Input: part model. Units: mm. Frame: model coordinates. Face numbers are marked on the shaded views. A direction names the side the tool comes from. Give positions to 0.01 mm unless a question says otherwise; leave off trailing zeros. Loops run counter-clockwise (first coordinate to the right, second up) from the corner with the lowest first, then second, coordinate; pieces in that order, holes last. Notation, with made-up numbers: M 27,53.5 L 63,53.5 A26 cw 63,70.5 Z; hole C 16.5,-19 d10. An arc over 180 degrees is marked long. Use CSV: the item, a comma, the result in double quotes. Start each with the question number.
Q1. Section D-D, the plane x = 29. Output: boundary loops of the cut face in (y, z), plus the area to 3 significant figures.
Q2. Reachability of the marked faces 1, 2, 3, 4 and 5 from +Z, -Z, +X, -X, +Y, -Y: full face, straight path, thin tool, end or side. Return the list, or none.
Q3. Pin query (flat end, axial travel): pin 1 (1.5 mm diameter, centred on x = 13, y = 65.5, fed in from +Z); pin 2 (5.5 mm diameter, centred on x = -23, z = 23, fed in from -Y); pin 3 (4 mm diameter, centred on y = 48, z = 26, fed in from +X). Return the tip coordinate at first contact, or that it passes through.
Q4. Section A-A, the plane y = 65. State how many separate pieces and enclosed holes the cut face has, plus the area to 3 significant figures.
Q5. Pull-direction query (Y, two-part tool) for the marked faces 6, 7, 8 and 9; classes: released by +Y, released by -Y, zero draft, split by the parting line, or undercut.
Q6. Section B-B, the plane x = -3. Output: boundary loops of the cut face in (y, z), plus the area to 3 significant figures.
Q7. Material intervals for line 1 along X through (y, z) = (24, 32); line 2 along Z through (x, y) = (28.5, 34); line 3 along X through (y, z) = (3.75, -23), sorted ascending.
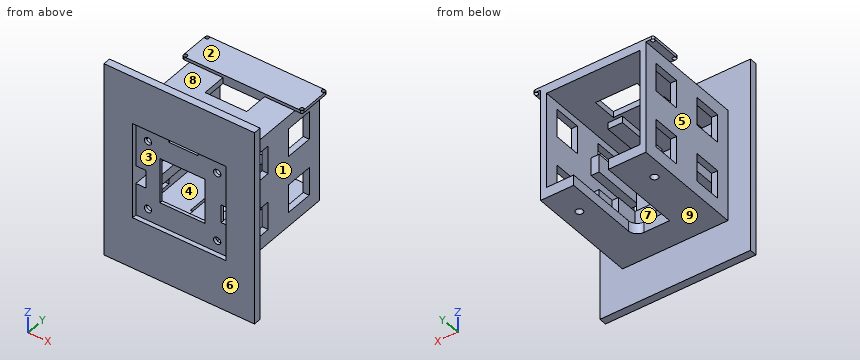
from build123d import *

# Parameters (mm, degrees)
SKETCH_1_W           = 100
SKETCH_1_H           = 130
EXTRUDE_1_DEPTH      = 5
SKETCH_2_W           = 70
SKETCH_2_H           = 75
SKETCH_2_W_2         = 62
SKETCH_2_H_2         = 64
EXTRUDE_2_DEPTH      = 73.5
SKETCH_3_W           = 18.75
SKETCH_3_H           = 18.4
CUT_EXTRUDE_1_DEPTH  = 133.711152508
CUT_EXTRUDE_2_DEPTH  = 10
SKETCH_7_W           = 62
SKETCH_7_H           = 64
CUT_EXTRUDE_3_DEPTH  = 3
SKETCH_8_W           = 30
SKETCH_8_H           = 30
CUT_EXTRUDE_4_DEPTH  = 3
SKETCH_9_R           = 2.4
CUT_EXTRUDE_5_DEPTH  = 112.468605446
SKETCH_11_W          = 14.189150171
SKETCH_11_H          = 10
EXTRUDE_3_DEPTH      = 18.5
SKETCH_12_W          = 4.351362518
SKETCH_12_H          = 10
EXTRUDE_4_DEPTH      = 33.5
SKETCH_13_W          = 6.623564314
SKETCH_13_H          = 6.911719061
SKETCH_13_H_2        = 12.024680345
SKETCH_13_W_2        = 5.320058298
SKETCH_13_W_3        = 8.691671684
SKETCH_13_H_3        = 4.310174588
SKETCH_13_W_4        = 9.602895329
EXTRUDE_5_DEPTH      = 33.5
SKETCH_14_R          = 2.4
CUT_EXTRUDE_6_DEPTH  = 40
EXTRUDE_8_DEPTH      = 2
SKETCH_21_R          = 1.25
CUT_EXTRUDE_9_DEPTH  = 2
SKETCH_22_W          = 27.664468573
SKETCH_22_H          = 16
CUT_EXTRUDE_10_DEPTH = 5
SKETCH_23_W          = 6.623564314
SKETCH_23_H          = 11.962590683
SKETCH_23_W_2        = 19.34597891
SKETCH_23_H_2        = 4.310174588
SKETCH_23_W_3        = 5.320058298
CUT_EXTRUDE_11_DEPTH = 111.123793978


with BuildPart() as part:
    # 草图1 → 凸台-拉伸1 (new body)
    with BuildSketch(Plane(origin=(0, 0, 0), x_dir=(1, 0, 0), z_dir=(0, 1, 0))):
        Rectangle(SKETCH_1_W, SKETCH_1_H)
    extrude(amount=EXTRUDE_1_DEPTH)

    # 草图2 → 凸台-拉伸2 (add)
    with BuildSketch(Plane(origin=(0, 5, 0), x_dir=(1, 0, 0), z_dir=(0, 1, 0))):
        with Locations((0, 0.285714286)):
            Rectangle(SKETCH_2_W, SKETCH_2_H)
        with Locations((0, -1.214285714)):
            Rectangle(SKETCH_2_W_2, SKETCH_2_H_2, mode=Mode.SUBTRACT)
    extrude(amount=EXTRUDE_2_DEPTH)

    # 草图3 → 切除-拉伸1 (cut, through all)
    with BuildSketch(Plane.ZY.offset(35)):
        with Locations((-19.035714286, 60.15)):
            Rectangle(SKETCH_3_W, SKETCH_3_H)
        with Locations((19.035714286, 60.15)):
            Rectangle(SKETCH_3_W, SKETCH_3_H)
        with Locations((19.035714286, 23.35)):
            Rectangle(SKETCH_3_W, SKETCH_3_H)
        with Locations((-19.035714286, 23.35)):
            Rectangle(SKETCH_3_W, SKETCH_3_H)
    extrude(amount=-CUT_EXTRUDE_1_DEPTH, mode=Mode.SUBTRACT)

    # 草图4 → 切除-拉伸2 (cut)
    with BuildSketch(Plane(origin=(0, 0, -37.785714286), x_dir=(-1, 0, 0), z_dir=(0, 0, -1))):
        with BuildLine():
            Line((-13, 78.5), (-13, 35.5))
            Line((-13, 35.5), (-13, 29.5))
            ThreePointArc((-13, 29.5), (-11.242640687, 25.257359313), (-7, 23.5))
            Line((-7, 23.5), (10, 23.5))
            Line((10, 23.5), (10, 78.5))
            Line((10, 78.5), (-13, 78.5))
        make_face()
    extrude(amount=-CUT_EXTRUDE_2_DEPTH, mode=Mode.SUBTRACT)

    # 草图7 → 切除-拉伸3 (cut)
    with BuildSketch(Plane(origin=(0, 0, 0), x_dir=(1, 0, 0), z_dir=(0, 1, 0))):
        with Locations((0, -1.214285714)):
            Rectangle(SKETCH_7_W, SKETCH_7_H)
    extrude(amount=CUT_EXTRUDE_3_DEPTH, mode=Mode.SUBTRACT)

    # 草图8 → 切除-拉伸4 (cut)
    with BuildSketch(Plane.XZ.offset(-3)):
        Rectangle(SKETCH_8_W, SKETCH_8_H)
    extrude(amount=-CUT_EXTRUDE_4_DEPTH, mode=Mode.SUBTRACT)

    # 草图9 → 切除-拉伸5 (cut, through all)
    with BuildSketch(Plane.XZ.offset(-3)):
        with Locations(Location((-23, -23, 0), (0, 0, 270))):
            Circle(SKETCH_9_R)
        with Locations(Location((23, -23, 0), (0, 0, 270))):
            Circle(SKETCH_9_R)
        with Locations(Location((23, 23, 0), (0, 0, 270))):
            Circle(SKETCH_9_R)
        with Locations(Location((-23, 23, 0), (0, 0, 270))):
            Circle(SKETCH_9_R)
    extrude(amount=-CUT_EXTRUDE_5_DEPTH, mode=Mode.SUBTRACT)

    # 草图11 → 凸台-拉伸3 (add)
    with BuildSketch(Plane(origin=(0, 5, 0), x_dir=(1, 0, 0), z_dir=(0, 1, 0))):
        with Locations((6.182659264, 25.785714286)):
            Rectangle(SKETCH_11_W, SKETCH_11_H)
    extrude(amount=EXTRUDE_3_DEPTH)

    # 草图12 → 凸台-拉伸4 (add)
    with BuildSketch(Plane(origin=(0, 5, 0), x_dir=(1, 0, 0), z_dir=(0, 1, 0))):
        with Locations((15.110555439, 25.785714286)):
            Rectangle(SKETCH_12_W, SKETCH_12_H)
    extrude(amount=EXTRUDE_4_DEPTH)

    # 草图13 → 凸台-拉伸5 (add)
    with BuildSketch(Plane(origin=(0, 5, 0), x_dir=(1, 0, 0), z_dir=(0, 1, 0))):
        with Locations((-27.688217843, 12.831804422)):
            Rectangle(SKETCH_13_W, SKETCH_13_H)
        with Locations((-27.688217843, -8.598985965)):
            Rectangle(SKETCH_13_W, SKETCH_13_H_2)
        with Locations((28.339970851, 12.831804422)):
            Rectangle(SKETCH_13_W_2, SKETCH_13_H)
        with Locations((28.339970851, -8.598985965)):
            Rectangle(SKETCH_13_W_2, SKETCH_13_H_2)
        with Locations((-13.432580878, -31.05919842)):
            Rectangle(SKETCH_13_W_3, SKETCH_13_H_3)
        with Locations((15.060681539, -31.05919842)):
            Rectangle(SKETCH_13_W_4, SKETCH_13_H_3)
    extrude(amount=EXTRUDE_5_DEPTH)

    # 草图14 → 切除-拉伸6 (cut)
    with BuildSketch(Plane(origin=(0, 0, -37.785714286), x_dir=(-1, 0, 0), z_dir=(0, 0, -1))):
        with Locations((-24.05892938, 58.5)):
            Circle(SKETCH_14_R)
        with Locations((25.94107062, 58.5)):
            Circle(SKETCH_14_R)
    extrude(amount=-CUT_EXTRUDE_6_DEPTH, mode=Mode.SUBTRACT)

    # 草图20 → 凸台-拉伸8 (add)
    with BuildSketch(Plane.XY.offset(37.214285714)):
        with BuildLine():
            Line((-38.7, 56.5), (38.7, 56.5))
            ThreePointArc((38.7, 56.5), (39.619238816, 56.880761184), (40, 57.8))
            Line((40, 57.8), (40, 77.2))
            ThreePointArc((40, 77.2), (39.619238816, 78.119238816), (38.7, 78.5))
            Line((38.7, 78.5), (-38.7, 78.5))
            ThreePointArc((-38.7, 78.5), (-39.619238816, 78.119238816), (-40, 77.2))
            Line((-40, 77.2), (-40, 57.8))
            ThreePointArc((-40, 57.8), (-39.619238816, 56.880761184), (-38.7, 56.5))
        make_face()
    extrude(amount=EXTRUDE_8_DEPTH)

    # 草图21 → 切除-拉伸9 (cut)
    with BuildSketch(Plane.XY.offset(39.214285714)):
        with Locations((-38.7, 77.2)):
            Circle(SKETCH_21_R)
        with Locations((-38.7, 57.8)):
            Circle(SKETCH_21_R)
        with Locations((38.7, 77.2)):
            Circle(SKETCH_21_R)
        with Locations((38.7, 57.8)):
            Circle(SKETCH_21_R)
    extrude(amount=-CUT_EXTRUDE_9_DEPTH, mode=Mode.SUBTRACT)

    # 草图22 → 切除-拉伸10 (cut)
    with BuildSketch(Plane.XY.offset(37.214285714)):
        with Locations((0.99347539, 48.5)):
            Rectangle(SKETCH_22_W, SKETCH_22_H)
    extrude(amount=-CUT_EXTRUDE_10_DEPTH, mode=Mode.SUBTRACT)

    # 草图23 → 切除-拉伸11 (cut, through all)
    with BuildSketch(Plane(origin=(0, 5, 0), x_dir=(1, 0, 0), z_dir=(0, 1, 0))):
        with Locations((-27.688217843, 3.39464955)):
            Rectangle(SKETCH_23_W, SKETCH_23_H)
        with Locations((0.586244419, -31.05919842)):
            Rectangle(SKETCH_23_W_2, SKETCH_23_H_2)
        with Locations((28.339970851, 3.39464955)):
            Rectangle(SKETCH_23_W_3, SKETCH_23_H)
    extrude(amount=-CUT_EXTRUDE_11_DEPTH, mode=Mode.SUBTRACT)


solid = part.part
A:
1,outline,"M 0,-65 L 5,-65 L 5,-37.79 L 78.5,-37.79 L 78.5,-30.79 L 5,-30.79 L 5,-16.29 L 38.5,-16.29 L 38.5,-9.38 L 3,-9.38 L 3,-30.79 L 0,-30.79 Z; M 0,33.21 L 3,33.21 L 3,2.59 L 38.5,2.59 L 38.5,14.61 L 5,14.61 L 5,33.21 L 78.5,33.21 L 78.5,39.21 L 56.5,39.21 L 56.5,37.21 L 5,37.21 L 5,65 L 0,65 Z"
1,area,"1,920 mm^2"
2,face 1,"-Z, +X, +Y"
2,face 2,"+Z, +X, -X, +Y"
2,face 3,"-Y"
2,face 4,"+Y"
2,face 5,"-Z, -X, +Y"
3,pin 1,"z = 39.21"
3,pin 2,"y = 3"
3,pin 3,"x = 35"
4,separate pieces,"5"
4,enclosed holes,"0"
4,area,"981 mm^2"
5,face 6,"released by -Y"
5,face 7,"released by +Y"
5,face 8,"undercut"
5,face 9,"zero draft"
6,outline,"M 0,-65 L 5,-65 L 5,-37.79 L 23.5,-37.79 L 23.5,-30.79 L 5,-30.79 L 5,-15 L 3,-15 L 3,-30.79 L 0,-30.79 Z; M 0,33.21 L 40.5,33.21 L 40.5,37.21 L 5,37.21 L 5,65 L 0,65 Z; M 3,15 L 5,15 L 5,28.9 L 3,28.9 Z; M 56.5,33.21 L 78.5,33.21 L 78.5,39.21 L 56.5,39.21 Z"
6,area,"793 mm^2"
7,line 1,"-35 to -31, -17.78 to -9.09, 10.26 to 19.86, 31 to 35"
7,line 2,"-37.79 to -30.79, -16.29 to -9.38, 2.59 to 14.61, 33.21 to 37.21"
7,line 3,"-50 to -25.4, -20.6 to 20.6, 25.4 to 50"
